```python
from build123d import *

# Parameters (mm, degrees)
F0_W     = 2070
F0_H     = 2036
F1_DEPTH = 3
F2_W     = 65
F2_H     = 65
F2_W_2   = 170
F2_H_2   = 170
F3_DEPTH = 6.001


with BuildPart() as f1:
    # F0 (on Top) → F1 (new body, symmetric)
    with BuildSketch(Plane.XY):
        Rectangle(F0_W, F0_H)
    extrude(amount=F1_DEPTH, both=True)

    # F2 (on face) → F3 (cut, through all)
    with BuildSketch(Plane.XY.offset(3)):
        with Locations((-1002.5, 985.5)):
            Rectangle(F2_W, F2_H)
        with Locations((-1035, 530)):
            Rectangle(F2_W_2, F2_H_2)
        with Locations((-1002.5, -985.5)):
            Rectangle(F2_W, F2_H)
        with Locations((-1035, -530)):
            Rectangle(F2_W_2, F2_H_2)
        with Locations((1002.5, 985.5)):
            Rectangle(F2_W, F2_H)
        with Locations((1002.5, -985.5)):
            Rectangle(F2_W, F2_H)
        with Locations((1035, -530)):
            Rectangle(F2_W_2, F2_H_2)
        with Locations((1035, 530)):
            Rectangle(F2_W_2, F2_H_2)
    extrude(amount=-F3_DEPTH, mode=Mode.SUBTRACT)


solid = f1.part
```
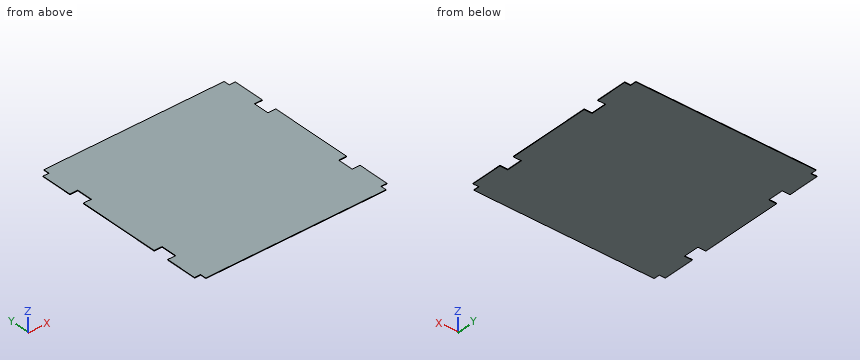
The listing builds one solid part. Answer for the finished solid, in the listing's coordinates (mm). Give positions to 0.01 mm unless a question says otherwise; leave off trailing zeros. Order: outer loops, then holes, each group sorted by start corner. A loop starts at its lowest first (then second) coordinate and runs counter-clockwise, first axis right, second up. Notation, with made-up numbers: M -16,22 L 36,22 A30 ccw 36,59 Z; hole C 73.25,86 d10. An arc over 180 degrees is marked long. Put each result on its own line as item: value. Start each with the question number.
Item 1: The part is cut by section A-A, the plane z = -0.7. Determine the outline of the cut face in (x, y), and give its area (3 significant figures).
Item 2: Flat-ended cylindrical pins translate along their axes: P1, Ø3, axis at y = 491, z = 1, coming from the +X side; P2, Ø1.8, axis at y = -981.5, z = 0, coming from the -X side; P3, Ø1.8, axis at x = -998.5, z = 0.5, coming from the +Y side. Find the tip coordinate at first contact, or state that the pin passes through.
Item 3: Find the intervals of material crossed by line 1 along Y through (x, z) = (-950.5, -2.2); line 2 along X through (y, z) = (-500, -2.7), in increasing order.
Item 4: The part is cut by section B-B, the plane y = -534. Determine the outline of the cut face in (x, z), and give its area (3 significant figures).
Answer key:
1. outline: M -1035,-953 L -970,-953 L -970,-1018 L 970,-1018 L 970,-953 L 1035,-953 L 1035,-615 L 950,-615 L 950,-445 L 1035,-445 L 1035,445 L 950,445 L 950,615 L 1035,615 L 1035,953 L 970,953 L 970,1018 L -970,1018 L -970,953 L -1035,953 L -1035,615 L -950,615 L -950,445 L -1035,445 L -1035,-445 L -950,-445 L -950,-615 L -1035,-615 Z
1. area: 4,140,000 mm²
2. P1: stops at x = 950
2. P2: stops at x = -970
2. P3: stops at y = 953
3. line 1: y = -1018 to -615, -445 to 445, 615 to 1018
3. line 2: x = -950 to 950
4. outline: M -950,-3 L 950,-3 L 950,3 L -950,3 Z
4. area: 11,400 mm²
